For this review, take the finished solid that the model builds, in its own axes (mm). Give positions to 0.01 mm unless a question says otherwise; leave off trailing zeros. Loops run counter-clockwise (first coordinate to the right, second up) from the corner with the lowest first, then second, coordinate; pieces in that order, holes last. Notation, with made-up numbers: (-27, -3) -> (-17, -3) arc R26 cw to (-17, 28) -> close; hole circle Ø1 at (-25.75, 85). An arc over 180 degrees is marked (long way). One line per question, with ' | ' between items. Start each with the question number.
(1) Consider section B-B (y = 9). Write out the cut boundary in (x, z).
(2) Wall thickness on probe 1 along Y at (x, z) = (16, -2.5); probe 2 along Z at (x, y) = (3, 6); probe 3 along X at (y, z) = (10, -4): over which ranges is each line inside the solid? List them lowest first.
(3) Draft analysis for pull direction X (two halves, no side actions). For faces 1 (the cylindrical face through (27.85, 9.126, -2.746)), 2 (the flat face through (18, 0, -4)), 3 (the flat face through (36.239, 9, -4)), state which applies: +X half, -X half, draft (parallel to the pull), parting line (faces both ways), or undercut.
(4) Consider section D-D (z = -6.25). Write out the cut boundary in (x, y).
(5) Consider section A-A (x = 29). Write out the cut boundary in (y, z), and give its area (3 significant figures).
(6) Consider section C-C (z = -4). Write out the cut boundary in (x, y), and give its area (3 significant figures).
(7) Insertion check: P1, Ø1.5, axis at y = 15, z = -3.5, coming from the -X side; P2, Ø6, axis at x = 16, y = 9, coming from the -Z side. Each pin has a flat end and moves straight along its axis. Give the tip position at first contact, or say it passes through.
Autodesk Inventor part; units mm, degrees
ref_plane "YZ Plane" through (0, 0, 0) normal (1, 0, 0) x (0, 1, 0)
ref_plane "XZ Plane" through (0, 0, 0) normal (0, 1, 0) x (-1, 0, 0)
ref_plane "XY Plane" through (0, 0, 0) normal (0, 0, 1) x (1, 0, 0)
sketch "Sketch1" plane through (0, 0, 0) normal (0, 1, 0) x (-1, 0, 0)
  line L0 (0, 0) -> (-32, 0)
  line L1 (-32, 0) -> (-32, -8)
  line L2 (-32, -8) -> (0, -8)
  line L3 (0, -8) -> (0, 0)
  line L4 (0, -4) -> (-32, -4) construction
  circle A0 centre (-3, -4) radius 1.5
  circle A1 centre (-29, -4) radius 1.5
  dimension "d1" = 8
  dimension "d2" = 26
  dimension "d20" = 3
  dimension "d21" = 3
  dimension "d22" = 3
extrude "Extrusion1" add sketch "Sketch1" along normal blind 18 contours L3 L2 L1 L0 | A0 | A1
hole "Hole1" at (29, 0, -4) at (3, 0, -4) direction (0, 1, 0) diameter 3.4036 end through all
sketch "Sketch2" plane through (0, 0, 0) normal (0, 0, 1) x (1, 0, 0)
  line L0 (0, 0) -> (32, 0)
  line L1 (32, 0) -> (32, 18)
  line L2 (0, 18) -> (32, 18)
  line L3 (0, 0) -> (0, 18)
  line L4 (0, 9) -> (32, 9)
  line L5 (32, 0) -> (32, 18)
  line L6 (16, 18) -> (16, 0)
  circle A0 centre (16, 9) radius 4.7625
  dimension "d28" = 9.525
hole "Hole2" at (16, 9, 0) direction (0, 0, -1) diameter 10.0838 end through all
sketch "Sketch3" plane through (32, 0, 0) normal (1, 0, 0) x (0, 0, -1)
  line L0 (0, 0) -> (8, 0)
  line L1 (8, 0) -> (8, 18)
  line L2 (0, 18) -> (8, 18)
  line L3 (0, 0) -> (0, 18)
  point P0 (0, 0)
extrude "Extrusion2" add sketch "Sketch3" along normal blind 4.239
equation "\"d22\" = d20"
properties part number "Drive Frame Tension Bearing Plate" material "Aluminum 6061"
A:
1) outline: (0, -8) -> (10.96, -8) -> (10.96, 0) -> (0, 0) -> close; (21.04, -8) -> (36.24, -8) -> (36.24, 0) -> (21.04, 0) -> close; hole circle Ø3.4 at (3, -4); hole circle Ø3.4 at (29, -4)
2) probe 1: y = 0 to 3.96, 14.04 to 18 | probe 2: z = -8 to -5.7, -2.3 to 0 | probe 3: x = 0 to 1.3, 4.7 to 11.06, 20.94 to 27.3, 30.7 to 36.24
3) face 1: undercut | face 2: draft | face 3: +X half
4) outline: (0, 0) -> (36.24, 0) -> (36.24, 18) -> (0, 18) -> close; hole circle Ø10.08 at (16, 9)
5) outline: (0, -8) -> (18, -8) -> (18, -5.7) -> (0, -5.7) -> close; (0, -2.3) -> (18, -2.3) -> (18, 0) -> (0, 0) -> close | area: 82.7 mm^2
6) outline: (0, 0) -> (1.3, 0) -> (1.3, 18) -> (0, 18) -> close; (4.7, 0) -> (27.3, 0) -> (27.3, 18) -> (4.7, 18) -> close; (30.7, 0) -> (36.24, 0) -> (36.24, 18) -> (30.7, 18) -> close; hole circle Ø10.08 at (16, 9) | area: 450 mm^2
7) P1: stops at x = 0 | P2: passes through
